```python
from build123d import *

# Parameters (mm, degrees)
F0_W     = 127
F0_H     = 327.025
F0_W_2   = 12.7
F1_DEPTH = 12.7
F3_D     = 6.7564


with BuildPart() as f1:
    # F0 (on Right) → F1 (new body)
    with BuildSketch(Plane.YZ):
        with Locations((-76.2, 176.2125)):
            Rectangle(F0_W, F0_H)
        with Locations((-6.35, 176.2125)):
            Rectangle(F0_W_2, F0_H)
    extrude(amount=F1_DEPTH)

    # F3 (through all)
    with Locations(Plane.YZ.offset(12.7)):
        with Locations((-127, 25.4), (-76.2, 25.4), (-25.4, 25.4)):
            Hole(F3_D / 2)


solid = f1.part
```
Geometry check sheet. Reference: the model listing, model coordinates, mm. Coordinates: 2 decimals unless noted, no trailing zeros. Loops run counter-clockwise (first coordinate to the right, second up) from the corner with the lowest first, then second, coordinate; pieces in that order, holes last.
Item 1: Sectioned sample at B-B, the plane z = 25.4. Record the boundary of the cut face in (x, y), then the cut area to 3 significant figures.
Item 2: Go/stop test with flat-tipped pins: pin 1 Ø8 at (y, z) = (-75.5, 265) entering from -X; pin 2 Ø6 at (y, z) = (-25.4, 25.4) entering from +X. Record where each tip stops, or that it passes through.
Item 3: Sectioned sample at A-A, the plane y = -76.2. Record the boundary of the cut face in (x, z) (3 decimals).
Item 4: Thickness scan on line 1 (Z direction, x = 7.75, y = -76.2) (3 decimals); line 2 (Z direction, x = 4, y = -130) (3 decimals). Record the ranges inside material, lowest first.
Item 5: Sectioned sample at C-C, the plane y = -25. Record the boundary of the cut face in (x, z) (3 decimals).
Item 6: Release check for a two-part mould opening along Y. For faces 1 (the face through (6, -139.7, 174)), 2 (the face through (0, -71, 179)), 3 (the face through (6.261, -130.222, 26.415)), 4 (the face through (6.261, -79.321, 24.106)) record: released by +Y, released by -Y, zero draft, split by the parting line, or undercut.
Check result:
1. outline: (0, -139.7) - (12.7, -139.7) - (12.7, -130.38) - (0, -130.38) - close; (0, -123.62) - (12.7, -123.62) - (12.7, -79.58) - (0, -79.58) - close; (0, -72.82) - (12.7, -72.82) - (12.7, -28.78) - (0, -28.78) - close; (0, -22.02) - (12.7, -22.02) - (12.7, 0) - (0, 0) - close
1. area: 1,520 mm2
2. pin 1: stops at x = 0
2. pin 2: passes through
3. outline: (0, 12.7) - (12.7, 12.7) - (12.7, 22.022) - (0, 22.022) - close; (0, 28.778) - (12.7, 28.778) - (12.7, 339.725) - (0, 339.725) - close
4. line 1: z = 12.7 to 22.022, 28.778 to 339.725
4. line 2: z = 12.7 to 23.847, 26.953 to 339.725
5. outline: (0, 12.7) - (12.7, 12.7) - (12.7, 22.046) - (0, 22.046) - close; (0, 28.754) - (12.7, 28.754) - (12.7, 339.725) - (0, 339.725) - close
6. face 1: released by -Y
6. face 2: zero draft
6. face 3: undercut
6. face 4: undercut
